Geometry: final body of the model. Coordinates: model frame, mm. A direction names the side the tool comes from. Give positions to 0.01 mm unless a question says otherwise; leave off trailing zeros. Write each loop counter-clockwise with the first axis right and the second up, starting at its lowest first coordinate (ties: lowest second). Pieces come first, ordered by that corner, then holes. Notation, with made-up numbers: (-23, -3.5) -> (27, -3.5) arc R25 cw to (27, 16.5) -> close; hole circle Ø2 at (-33.5, 30). An arc over 180 degrees is marked (long way). Answer in a Markdown table with one row per item. Add a question column.
Item 1: Section query C-C on x = -1.45. Output: boundary loops of the cut face in (y, z), plus the area to 3 significant figures.
Item 2: Material intervals for probe 1 along X at (y, z) = (-2.25, 0.55); probe 2 along Y at (x, z) = (0.05, -0.5); probe 3 along Y at (x, z) = (-1.35, 0.2), sorted ascending. Write a range as from..to.
Item 3: Section query A-A on y = 1. Output: boundary loops of the cut face in (x, z).
Item 4: Section query B-B on z = 0. Output: boundary loops of the cut face in (x, y), plus the area to 3 significant figures.
Item 5: Section query D-D on y = -2. Output: boundary loops of the cut face in (x, z), plus the area to 3 significant figures.
Item 6: Access query for faces 1 (the flat face through (-1.95, 0, 0)), 2 (the cylindrical face through (-1.34, 0.27, -1.22)). Directions: +Z, -Z, +X, -X, +Y, -Y. A direction counts if a zero-diameter tool reaches every point of the face in a straight line with its end or side. Return the directions, or none.
```python
from build123d import *

# Parameters (mm, degrees)
F1_DEPTH = 0.75
F2_R     = 0.5
F3_R     = 1.25
F4_DEPTH = 1.2


with BuildPart() as f1:
    # F0 (on Right) → F1 (new body, symmetric)
    with BuildSketch(Plane.YZ):
        with BuildLine():
            Line((2.5, 1.25), (-2.5, 1.25))
            ThreePointArc((-2.5, 1.25), (-3.75, 0), (-2.5, -1.25))
            Line((-2.5, -1.25), (2.5, -1.25))
            ThreePointArc((2.5, -1.25), (3.75, 0), (2.5, 1.25))
        make_face()
    extrude(amount=F1_DEPTH, both=True)

    # F2
    f2_edges = [f1.edges().sort_by_distance(p)[0] for p in [
        (0.75, 0, 1.25),
        (0.75, -3.75, 0),
        (0.75, 0, -1.25),
        (0.75, 3.75, 0),
    ]]
    fillet(f2_edges, radius=F2_R)

    # F3 (on face) → F4 (join)
    with BuildSketch(Plane(origin=(-0.75, 0, 0), x_dir=(0, -1, 0), z_dir=(-1, 0, 0))):
        Circle(F3_R)
    extrude(amount=F4_DEPTH)


solid = f1.part
```
Findings below:
| question | item | result |
|---|---|---|
| 1 | outline | circle Ø2.5 at (0, 0) |
| 1 | area | 4.91 mm^2 |
| 2 | probe 1 | x = -0.75..0.75 |
| 2 | probe 2 | y = -3.65..3.65 |
| 2 | probe 3 | y = -1.23..1.23 |
| 3 | outline | (-1.95, -0.75) -> (-0.75, -0.75) -> (-0.75, -1.25) -> (0.25, -1.25) arc R0.5 ccw to (0.75, -0.75) -> (0.75, 0.75) arc R0.5 ccw to (0.25, 1.25) -> (-0.75, 1.25) -> (-0.75, 0.75) -> (-1.95, 0.75) -> close |
| 4 | outline | (-1.95, -1.25) -> (-0.75, -1.25) -> (-0.75, -3.75) -> (0.25, -3.75) arc R0.5 ccw to (0.75, -3.25) -> (0.75, 3.25) arc R0.5 ccw to (0.25, 3.75) -> (-0.75, 3.75) -> (-0.75, 1.25) -> (-1.95, 1.25) -> close |
| 4 | area | 14.1 mm^2 |
| 5 | outline | (-0.75, -1.25) -> (0.25, -1.25) arc R0.5 ccw to (0.75, -0.75) -> (0.75, 0.75) arc R0.5 ccw to (0.25, 1.25) -> (-0.75, 1.25) -> close |
| 5 | area | 3.64 mm^2 |
| 6 | face 1 | +Z, -Z, -X, +Y, -Y |
| 6 | face 2 | -X |
